from build123d import *

# Parameters (mm, degrees)
SKETCH1_R            = 8.5
BOSS_EXTRUDE1_DEPTH  = 17
SKETCH2_R            = 10.5
BOSS_EXTRUDE2_DEPTH  = 10
CHAMFER1_SIZE        = 5.494954839
CHAMFER1_SIZE_2      = 2
SKETCH3_R            = 8.5
CUT_EXTRUDE1_DEPTH   = 1
SKETCH4_R            = 9.5
BOSS_EXTRUDE3_DEPTH  = 15
SKETCH9_W            = 11
SKETCH9_H            = 11
BOSS_EXTRUDE4_DEPTH  = 3
SKETCH10_W           = 2
SKETCH10_H           = 5
BOSS_EXTRUDE5_DEPTH  = 7
FILLET1_R            = 2.5
SKETCH13_R           = 8.4
BOSS_EXTRUDE7_DEPTH  = 1.5
FILLET3_R            = 7
SKETCH14_W           = 5
SKETCH14_H           = 12
BOSS_EXTRUDE9_DEPTH  = 2
SKETCH15_W           = 5
SKETCH15_H           = 11.75
BOSS_EXTRUDE10_DEPTH = 2
FILLET4_START        = -5.5
FILLET4_DEPTH        = 4.5
FILLET4_START_2      = 1
FILLET4_2_DEPTH      = 4.5
CUT_EXTRUDE3_REACH   = 51.064
SKETCH16_R           = 0.875


with BuildPart() as part:
    # Sketch1 → Boss-Extrude1 (new body)
    with BuildSketch(Plane.XY):
        Circle(SKETCH1_R)
    extrude(amount=-BOSS_EXTRUDE1_DEPTH)

    # Sketch2 → Boss-Extrude2 (add)
    with BuildSketch(Plane.XY):
        Circle(SKETCH2_R)
    extrude(amount=BOSS_EXTRUDE2_DEPTH)

    # Chamfer1
    # the kernel refuses this chamfer: 5.494954839, 2 mm, written as the material it takes off along each edge
    with BuildSketch(Plane(origin=(0, 0, 0), x_dir=(1, 0, 0), z_dir=(0, -1, 0))) as chamfer1_piece_1_section:
        Polygon((10.5, CHAMFER1_SIZE), (10.5 - CHAMFER1_SIZE_2, 0), (10.5, 0), align=None)
    chamfer1_piece_1 = revolve(axis=Axis((0, 0, 0), (0, 0, 1)), mode=Mode.PRIVATE)
    chamfer1_piece_1 = chamfer1_piece_1 - Plane(origin=(0, 0, 0), x_dir=(1, 0, 0), z_dir=(0, 0, 1)) * Cylinder(8.5, 42, mode=Mode.PRIVATE)
    add(chamfer1_piece_1, mode=Mode.SUBTRACT)

    # Sketch3 → Cut-Extrude1 (cut)
    with BuildSketch(Plane.XY.offset(10)):
        Circle(SKETCH3_R)
    extrude(amount=-CUT_EXTRUDE1_DEPTH, mode=Mode.SUBTRACT)

    # Sketch4 → Boss-Extrude3 (add)
    with BuildSketch(Plane(origin=(0, 0, -17), x_dir=(-1, 0, 0), z_dir=(0, 0, -1))):
        Circle(SKETCH4_R)
    extrude(amount=BOSS_EXTRUDE3_DEPTH)

    # Loft2: read off the stored shape, not the designer's step
    # Loft2: loft between two sections, ruled curve by curve
    loft2_from = [
        Edge.make_bspline([(5.6816796, 5.631919471, -32), (16.945518542, -5.731439728, -32), (5.582159343, -16.99527867, -32), (-5.6816796, -5.631919471, -32), (-16.945518542, 5.731439728, -32), (-5.582159343, 16.99527867, -32), (5.6816796, 5.631919471, -32)], [0, 0, 0, 0, 0.5, 0.5, 0.5, 1, 1, 1, 1], 3, [1, 0.333333333, 0.333333333, 1, 0.333333333, 0.333333333, 1]),
    ]
    loft2_to = [
        Edge.make_bspline([(2.275915377, 1.034509157, -40), (4.344933691, -3.517321597, -40), (-0.206897063, -5.586339911, -40), (-2.275915377, -1.034509157, -40), (-4.344933691, 3.517321597, -40), (0.206897063, 5.586339911, -40), (2.275915377, 1.034509157, -40)], [0, 0, 0, 0, 0.5, 0.5, 0.5, 1, 1, 1, 1], 3, [1, 0.333333333, 0.333333333, 1, 0.333333333, 0.333333333, 1]),
    ]
    loft2 = Solid(Shell([*[Face.make_surface_from_curves(loft2_from[k], loft2_to[k]) for k in range(1)], Face(Wire(loft2_from)), Face(Wire(loft2_to))]))
    add(loft2)

    # Sketch9 → Boss-Extrude4 (add)
    with BuildSketch(Plane(origin=(0, -8, 0), x_dir=(1, 0, 0), z_dir=(0, 1, 0))):
        with Locations((0, 24.5)):
            Rectangle(SKETCH9_W, SKETCH9_H)
    extrude(amount=-BOSS_EXTRUDE4_DEPTH)

    # Sketch10 → Boss-Extrude5 (add)
    with BuildSketch(Plane.XZ.offset(11)):
        with Locations((0, -21.5)):
            Rectangle(SKETCH10_W, SKETCH10_H)
    extrude(amount=BOSS_EXTRUDE5_DEPTH)

    # Fillet1
    fillet1_edges = [part.edges().sort_by_distance(p)[0] for p in [
        (0, -18, -19),
        (0, -18, -24),
    ]]
    fillet(fillet1_edges, radius=FILLET1_R - 0.0001)  # a hair under: the kernel refuses the full size

    # Sketch13 → Boss-Extrude7 (add)
    with BuildSketch(Plane.XY.offset(9)):
        Circle(SKETCH13_R)
    extrude(amount=BOSS_EXTRUDE7_DEPTH)

    # Fillet3
    # the kernel refuses this fillet: 7 mm, written as the material it takes off along each edge
    with BuildSketch(Plane(origin=(0, 0, 10.5), x_dir=(1, 0, 0), z_dir=(0, -1, 0))) as fillet3_piece_1:
        with BuildLine():
            CenterArc((4.069872981, -7), FILLET3_R, 51.786789298, 38.213210702)
            Line((4.069872981, 0), (8.4, 0))
            Line((8.4, 0), (8.4, -1.5))
        make_face()
    revolve(axis=Axis((0, 0, 10.5), (0, 0, 1)), mode=Mode.SUBTRACT)

    # Sketch14 → Boss-Extrude9 (add)
    with BuildSketch(Plane(origin=(1, 0, 0), x_dir=(0, 0, -1), z_dir=(1, 0, 0))):
        with Locations((21.5, -19)):
            Rectangle(SKETCH14_W, SKETCH14_H)
    extrude(amount=BOSS_EXTRUDE9_DEPTH)

    # Sketch15 → Boss-Extrude10 (add)
    with BuildSketch(Plane.ZY.offset(1)):
        with Locations((-21.5, -19.125)):
            Rectangle(SKETCH15_W, SKETCH15_H)
    extrude(amount=BOSS_EXTRUDE10_DEPTH)

    # Fillet4: read off the stored shape, not the designer's step
    # Fillet4 outline → Fillet4 (cut)
    with BuildSketch(Plane.YZ.offset(FILLET4_START)):
        with BuildLine():
            Line((-25, -19), (-25, -21.5))
            ThreePointArc((-25, -21.5), (-24.267766953, -19.732233047), (-22.5, -19))
            Line((-22.5, -19), (-25, -19))
        make_face()
        with BuildLine():
            ThreePointArc((-22.5, -24), (-24.267766953, -23.267766953), (-25, -21.5))
            Line((-25, -21.5), (-25, -24))
            Line((-25, -24), (-22.5, -24))
        make_face()
        with BuildLine():
            ThreePointArc((-13.25, -21.5), (-13.982233047, -23.267766953), (-15.75, -24))
            Line((-15.75, -24), (-13.25, -24))
            Line((-13.25, -24), (-13.25, -21.5))
        make_face()
        with BuildLine():
            ThreePointArc((-15.75, -19), (-13.982233047, -19.732233047), (-13.25, -21.5))
            Line((-13.25, -21.5), (-13.25, -19))
            Line((-13.25, -19), (-15.75, -19))
        make_face()
    extrude(amount=FILLET4_DEPTH, mode=Mode.SUBTRACT)

    # Fillet4 2 outline → Fillet4 2 (cut)
    with BuildSketch(Plane.YZ.offset(FILLET4_START_2)):
        with BuildLine():
            Line((-25, -19), (-25, -21.5))
            ThreePointArc((-25, -21.5), (-24.267766953, -19.732233047), (-22.5, -19))
            Line((-22.5, -19), (-25, -19))
        make_face()
        with BuildLine():
            ThreePointArc((-22.5, -24), (-24.267766953, -23.267766953), (-25, -21.5))
            Line((-25, -21.5), (-25, -24))
            Line((-25, -24), (-22.5, -24))
        make_face()
        with BuildLine():
            Line((-15.5, -24), (-13, -24))
            Line((-13, -24), (-13, -21.5))
            ThreePointArc((-13, -21.5), (-13.732233047, -23.267766953), (-15.5, -24))
        make_face()
        with BuildLine():
            ThreePointArc((-15.5, -19), (-13.732233047, -19.732233047), (-13, -21.5))
            Line((-13, -21.5), (-13, -19))
            Line((-13, -19), (-15.5, -19))
        make_face()
    extrude(amount=FILLET4_2_DEPTH, mode=Mode.SUBTRACT)

    # Cut-Extrude3: up to this face of the body (flat: up to its plane)
    cut_extrude3_end = Plane(part.part.faces().sort_by_distance((3, -19, -21.5))[0])
    # Sketch16 → Cut-Extrude3 (cut, up to the picked face)
    with BuildSketch(Plane.ZY.offset(3), mode=Mode.PRIVATE) as cut_extrude3_sk1:
        with Locations((-21.5, -15.75)):
            Circle(SKETCH16_R)
    cut_extrude3_tool1 = split(extrude(cut_extrude3_sk1.sketch, amount=-CUT_EXTRUDE3_REACH, mode=Mode.PRIVATE), bisect_by=cut_extrude3_end, keep=Keep.BOTH, mode=Mode.PRIVATE)
    # Sketch16 → Cut-Extrude3 (cut, up to the picked face)
    with BuildSketch(Plane.ZY.offset(3), mode=Mode.PRIVATE) as cut_extrude3_sk2:
        with Locations((-21.5, -22.5)):
            Circle(SKETCH16_R)
    cut_extrude3_tool2 = split(extrude(cut_extrude3_sk2.sketch, amount=-CUT_EXTRUDE3_REACH, mode=Mode.PRIVATE), bisect_by=cut_extrude3_end, keep=Keep.BOTH, mode=Mode.PRIVATE)
    add(cut_extrude3_tool1.solids().sort_by(Axis((-3, -15.75, -21.5), (1, 0, 0)))[0], mode=Mode.SUBTRACT)
    add(cut_extrude3_tool2.solids().sort_by(Axis((-3, -22.5, -21.5), (1, 0, 0)))[0], mode=Mode.SUBTRACT)


solid = part.part
Part model, mm, in its own coordinate system. A direction names the side the tool comes from. Round coordinates to 2 decimals unless told otherwise and drop trailing zeros. Order: outer loops, then holes, each group sorted by start corner. A loop starts at its lowest first (then second) coordinate and runs counter-clockwise, first axis right, second up. Notation, with made-up numbers: (55, 25.5) -> (78, 25.5) arc R15 cw to (78, 52.5) -> close; hole circle Ø6 at (8.25, 20). An arc over 180 degrees is marked (long way). Put each result on its own line as item: value.
Q1. Tool access for faces 5 (the face through (3, -19, -21)), 6 (the face through (5.5, -9, -24)), 7 (the face through (-5.5, -9, -24)), 8 (the face through (10, 3.2, 7.7)): list every direction of +Z, -Z, +X, -X, +Y, -Y with a clear straight run to the whole face (end or side of a thin tool).
From the geometry:
face 5: +Z, -Z, +X, -Y
face 6: -Z, +X, -Y
face 7: -Z, -X, -Y
face 8: +Z
Q2. Band-saw the part on A-A (y = -19.5). Give the cut face in (x, z).
From the geometry:
outline: (-3, -24) -> (-1, -24) -> (-1, -19) -> (-3, -19) -> close; (1, -24) -> (3, -24) -> (3, -19) -> (1, -19) -> close
Q3. Pull direction Z, two halves, no side cores. Call faces 1 (the face through (-2, -19, -19)), 2 (the face through (2.2, -8.4, -17)), 3 (the face through (1.99, -23.28, -21.1)), 4 (the face through (1.5, -16.8, -24)): pulls with the +Z half, pulls with the -Z half, needs draft (parallel to the pull), parting line crosses it, or undercut.
From the geometry:
face 1: pulls with the +Z half
face 2: undercut
face 3: undercut
face 4: pulls with the -Z half
Q4. Pin check, flat tips, straight feed: pin 1 Ø1.4 at (y, z) = (-12.5, -22.5) entering from -X; pin 2 Ø12 at (y, z) = (-19.5, -18.5) entering from +X; pin 3 Ø1.5 at (y, z) = (-19, -22) entering from -X. Stop position of each tip, or through.
From the geometry:
pin 1: stops at x = -1
pin 2: stops at x = 3
pin 3: stops at x = -3
Q5. Band-saw the part on B-B (z = -5). Give the cut face in (x, y).
From the geometry:
outline: circle Ø17 at (0, 0)
Q6. Wall check: line 1 (Y direction, x = -0.4, z = -21.5) (3 decimals); line 2 (X direction, y = -13, z = -22); line 3 (X direction, y = -9.5, z = -29). Give the ranges that are in metal, low to high. Write a range as [from, to].
From the geometry:
line 1: y = [-18, -16.625], [-14.875, 9.492]
line 2: x = [-1, 1]
line 3: x = [-5.5, 5.5]
